The listing builds one solid part. Answer for the finished solid, in the listing's coordinates (mm). A direction names the side the tool comes from. Coordinates: 2 decimals unless noted, no trailing zeros. Order: outer loops, then holes, each group sorted by start corner. A loop starts at its lowest first (then second) coordinate and runs counter-clockwise, first axis right, second up. Notation, with made-up numbers: (24, 18.25) -> (54, 18.25) arc R22 ccw to (54, 29.25) -> close; hole circle Ø9 at (17.5, 37.5). An arc over 180 degrees is marked (long way). Put each result on its own line as item: value. Start each with the question number.
```python
from build123d import *

# Parameters (mm, degrees)
EXTRUDE_DEPTH           = 10
EXTRUDE_PLACEMENT_ANGLE = 270
CYLINDER004_R           = 34
CYLINDER004_DEPTH       = 30
CYLINDER003_R           = 4
CYLINDER003_DEPTH       = 120
CYLINDER005_R           = 20
CYLINDER005_DEPTH       = 20
CYLINDER_R              = 46
CYLINDER_DEPTH          = 60


with BuildPart() as extrude_body:
    # path2399 → Extrude (new body)
    with BuildSketch(Plane(origin=(8.682374, 337.01873, 81), x_dir=(0, 1, 0), z_dir=(0, 0, 1))):
        with BuildLine():
            add(Edge.make_bspline(
                [(-1.415579, 5.024931), (-1.938341, -2.484397)],
                knots=[0, 0, 7.527502, 7.527502], degree=1))
            add(Edge.make_bspline(
                [(-1.938341, -2.484397), (-1.938341, -2.484397), (-2.134903, -2.858259), (-2.273136, -3.334737)],
                knots=[0, 0, 0, 0, 1, 1, 1, 1], degree=3))
            add(Edge.make_bspline(
                [(-2.273136, -3.334737), (-2.411369, -3.811216), (-2.443203, -4.128926), (-2.371685, -4.540758)],
                knots=[0, 0, 0, 0, 1, 1, 1, 1], degree=3))
            add(Edge.make_bspline(
                [(-2.371685, -4.540758), (-2.300167, -4.952591), (-2.218933, -5.672599), (-1.772797, -6.040394)],
                knots=[0, 0, 0, 0, 1, 1, 1, 1], degree=3))
            add(Edge.make_bspline(
                [(-1.772797, -6.040394), (-1.326661, -6.40819), (-0.861351, -6.572675), (-0.583202, -6.662312)],
                knots=[0, 0, 0, 0, 1, 1, 1, 1], degree=3))
            add(Edge.make_bspline(
                [(-0.583202, -6.662312), (-0.305053, -6.751952), (0.507781, -6.731952), (0.709843, -6.630052)],
                knots=[0, 0, 0, 0, 1, 1, 1, 1], degree=3))
            add(Edge.make_bspline(
                [(0.709843, -6.630052), (0.911905, -6.52815), (1.481843, -6.245909), (1.726833, -5.892641)],
                knots=[0, 0, 0, 0, 1, 1, 1, 1], degree=3))
            add(Edge.make_bspline(
                [(1.726833, -5.892641), (1.971823, -5.539373), (2.340182, -5.059724), (2.384256, -4.759981)],
                knots=[0, 0, 0, 0, 1, 1, 1, 1], degree=3))
            add(Edge.make_bspline(
                [(2.384256, -4.759981), (2.42833, -4.460237), (2.223091, -3.691858), (2.158411, -3.465999)],
                knots=[0, 0, 0, 0, 1, 1, 1, 1], degree=3))
            add(Edge.make_bspline(
                [(2.158411, -3.465999), (2.093732, -3.240141), (1.863634, -2.929328), (1.863634, -2.929328)],
                knots=[0, 0, 0, 0, 1, 1, 1, 1], degree=3))
            add(Edge.make_bspline(
                [(1.863634, -2.929328), (1.423808, 5.709855)],
                knots=[0, 0, 8.650371, 8.650371], degree=1))
            add(Edge.make_bspline(
                [(1.423808, 5.709855), (1.423808, 5.709855), (1.246198, 6.226563), (0.794563, 6.495307)],
                knots=[0, 0, 0, 0, 1, 1, 1, 1], degree=3))
            add(Edge.make_bspline(
                [(0.794563, 6.495307), (0.342929, 6.764051), (-0.057622, 6.753041), (-0.37358, 6.666974)],
                knots=[0, 0, 0, 0, 1, 1, 1, 1], degree=3))
            add(Edge.make_bspline(
                [(-0.37358, 6.666974), (-0.689538, 6.580907), (-1.208145, 6.230265), (-1.306201, 5.897514)],
                knots=[0, 0, 0, 0, 1, 1, 1, 1], degree=3))
            add(Edge.make_bspline(
                [(-1.306201, 5.897514), (-1.404257, 5.564763), (-1.415579, 5.024931), (-1.415579, 5.024931)],
                knots=[0, 0, 0, 0, 1, 1, 1, 1], degree=3))
        make_face()
    extrude(amount=EXTRUDE_DEPTH)


with BuildPart() as extrude_body_1:
    # Extrude placement: moved
    add(extrude_body.part.moved(Location((-13, -13, 406))).rotate(Axis((-13, -13, 406), (1, 0, 0)), EXTRUDE_PLACEMENT_ANGLE))


with BuildPart() as cylinder004:
    # Cylinder004 → Cylinder004 (new body)
    with BuildSketch(Plane.XY.offset(56)):
        Circle(CYLINDER004_R)
    extrude(amount=CYLINDER004_DEPTH)


with BuildPart() as cut:
    # Cylinder003 → Cylinder003 (new body)
    with BuildSketch(Plane(origin=(0, 60, 70), x_dir=(1, 0, 0), z_dir=(0, -1, 0))):
        Circle(CYLINDER003_R)
    extrude(amount=CYLINDER003_DEPTH)

    # Cut: cut Cylinder004
    add(cylinder004.part, mode=Mode.SUBTRACT)


with BuildPart() as cut001:
    # Cylinder005 → Cylinder005 (new body)
    with BuildSketch(Plane(origin=(0, 70, 70), x_dir=(1, 0, 0), z_dir=(0, -1, 0))):
        Circle(CYLINDER005_R)
    extrude(amount=CYLINDER005_DEPTH)

    # Fusion: union Cut
    add(cut.part)

    # Cut001: cut Extrude body
    add(extrude_body_1.part, mode=Mode.SUBTRACT)


with BuildPart() as cylinder:
    # Cylinder → Cylinder (new body)
    with BuildSketch(Plane.XY):
        Circle(CYLINDER_R)
    extrude(amount=CYLINDER_DEPTH)


with BuildPart() as fusion001:
    # Sketch → Revolve (revolve)
    with BuildSketch(Plane.XZ):
        Polygon((0, 1), (34, 1), (34, 70), (38, 70), (38, 0), (0, 0), align=None)
    revolve(axis=Axis((0, 0, 0), (0, 0, 1)))

    # Cut002: cut Cylinder
    add(cylinder.part, mode=Mode.SUBTRACT)

    # Fusion001: union Cut001
    add(cut001.part)


solid = fusion001.part
```
(1) The part is cut by section D-D on y = 57.5. Determine the outline of the cut face in (x, z).
(2) Find the intervals of material crossed by L1, parallel to Y at x = 0, z = 63; L2, parallel to X at y = 0, z = 68; L3, parallel to Y at x = 0, z = 66.5, in increasing order.
(3) The part is cut by section A-A on y = 0. Determine the outline of the cut face in (x, z), plus the area to 3 significant figures.
(4) A tool of negligible diameter and unlimited length cuts with its end or side. For faces 1 (the cylindrical face through (32.43, 10.21, 63.81)), 2 (the flat face through (-34, 6, 70)), 3 (the flat face through (-28, -20, 60)), 4 (the cylindrical face through (-0.521, -46.698, 73.966)), from which of +Z, -Z, +X, -X, +Y, -Y can it reach the whole face along a straight path? Write none if from no direction.
(5) Each of these flat-tipped pins is pushed along its axis until it touches: P1, Ø1, axis at x = -7.5, z = 60.5, coming from the -Y side; P2, Ø3, axis at x = 10.5, z = 77, coming from the -Y side; P3, Ø2.5, axis at x = -6.5, z = 68, coming from the +Y side. Where does it stop, or does it pass through?
(6) The part is cut by section B-B on x = 32. Determine the outline of the cut face in (y, z).
(7) For a pull along Y with two mould halves and no side action, classify faces 5 (the flat face through (35, 0, 70)), 6 (the flat face through (0, -60, 70)), 7 (the cylindrical face through (-0.521, 41.996, 73.966)) as released by +Y, released by -Y, zero draft, split by the parting line, or undercut.
(8) The part is cut by section C-C on z = 82. Determine the outline of the cut face in (x, y).
Worked out:
1. outline: circle Ø40 at (0, 70)
2. L1: -38 to -34, 34 to 38, 50 to 70
2. L2: -38 to -34, 34 to 38
2. L3: -60 to -34, 34 to 70
3. outline: (-38, 60) -> (-34, 60) -> (-34, 70) -> (-38, 70) -> close; (34, 60) -> (38, 60) -> (38, 70) -> (34, 70) -> close
3. area: 80.0 mm2
4. face 1: +Z, -Z
4. face 2: +Z, -X, -Y
4. face 3: -Z, +X, -X, -Y
4. face 4: -Y
5. P1: y = -37.35
5. P2: y = 50
5. P3: y = 70
6. outline: (-20.49, 60) -> (-11.49, 60) -> (-11.49, 70) -> (-20.49, 70) -> close; (11.49, 60) -> (20.49, 60) -> (20.49, 70) -> (11.49, 70) -> close
7. face 5: zero draft
7. face 6: released by -Y
7. face 7: undercut
8. outline: (-16, 50) -> (16, 50) -> (16, 70) -> (-16, 70) -> close
